```python
from build123d import *

# Parameters (mm, degrees)
F2_W           = 1
F2_H           = 12
F4_R           = 1.9571428571
F7_START       = 17.5
F7_DEPTH       = 42.5
F11_R          = 6
F12_DEPTH      = 25
F12_DEPTH_BACK = 25


with BuildPart() as f1:
    # F0 (on Front) → F1 (revolve)
    with BuildSketch(Plane.XZ):
        with BuildLine():
            Line((-199.1, 17.5), (-199.1, 0))
            Line((-199.1, 0), (75.9, 0))
            Line((75.9, 0), (75.9, 12.5))
            Line((75.9, 12.5), (70.9, 17.5))
            Line((70.9, 17.5), (26.1, 17.5))
            Line((26.1, 17.5), (26.1, 22.5))
            Line((26.1, 22.5), (22.4, 22.5))
            ThreePointArc((22.4, 22.5), (19.5715728753, 23.6715728753), (18.4, 26.5))
            Line((18.4, 26.5), (18.4, 30))
            Line((18.4, 30), (0, 30))
            Line((0, 30), (0, 22.5))
            Line((0, 22.5), (-69.7, 22.5))
            Line((-69.7, 22.5), (-69.7, 17.5))
            Line((-69.7, 17.5), (-199.1, 17.5))
        make_face()
    revolve(axis=Axis((-55.8219029194, 0, 0), (1, 0, 0)))

    # F2 (on Front) → F3 (revolve, cut)
    with BuildSketch(Plane.XZ):
        with Locations((-50.5, 27.5)):
            Rectangle(F2_W, F2_H)
    revolve(axis=Axis((-55.8219029194, 0, 0), (1, 0, 0)), mode=Mode.SUBTRACT)

    # F4 (on Front) → F5 (revolve, cut)
    with BuildSketch(Plane.XZ):
        with Locations((-86.2, 18.7571428571)):
            Circle(F4_R)
        with Locations((42.6, 18.7571428571)):
            Circle(F4_R)
        with BuildLine():
            Line((-3.4571428571, 32.4009352645), (-3.4571428571, 23.7571428571))
            ThreePointArc((-3.4571428571, 23.7571428571), (-2.1688399949, 21.9178328712), (0, 22.5))
            Line((0, 22.5), (0, 32.4009352645))
            Line((0, 32.4009352645), (-3.4571428571, 32.4009352645))
        make_face()
    revolve(axis=Axis((-55.8219029194, 0, 0), (1, 0, 0)), mode=Mode.SUBTRACT)

    # F6 (on Top) → F7 (cut)
    with BuildSketch(Plane.XY.offset(F7_START)):
        with BuildLine():
            Line((-9, 5), (-39, 5))
            ThreePointArc((-39, 5), (-44, 0), (-39, -5))
            Line((-39, -5), (-9, -5))
            ThreePointArc((-9, -5), (-4, 0), (-9, 5))
        make_face()
    extrude(amount=F7_DEPTH, mode=Mode.SUBTRACT)

    # F11 (on line) → F12 (cut, two sides)
    with BuildSketch(Plane(origin=(0, 0, 0), x_dir=(1, 0, 0), z_dir=(0, -0.8660254038, -0.5))) as f12_sk:
        with Locations((-149.1, 0)):
            Circle(F11_R)
    extrude(amount=-F12_DEPTH, mode=Mode.SUBTRACT)
    extrude(f12_sk.sketch, amount=F12_DEPTH_BACK, mode=Mode.SUBTRACT)


solid = f1.part
```
Input: part model. Units: mm. Frame: model coordinates. A direction names the side the tool comes from. Coordinates: 2 decimals unless noted, no trailing zeros. Write each loop counter-clockwise with the first axis right and the second up, starting at its lowest first coordinate (ties: lowest second). Pieces come first, ordered by that corner, then holes. Notation, with made-up numbers: (-14, 81.25) - (10, 81.25) arc R17 cw to (10, 111.25) - close; hole circle Ø2 at (36.25, 16.25). An arc over 180 degrees is marked (long way). Put each result on its own line as item: value. Start each with the question number.
1) Contact query for flat-ended pins moving along their axis: pin 1 (10 mm diameter, centred on x = -14.5, z = 4, fed in from +Y); pin 2 (5 mm diameter, centred on x = -10, y = -12.5, fed in from +Z); pin 3 (8 mm diameter, centred on x = 37, y = 22, fed in from +Z); pin 4 (6 mm diameter, centred on x = -168, z = -9, fed in from -Y). Output: stop coordinate, or through.
2) Reachability of faces 1 (the face through (-24, 5, 20)), 2 (the face through (26.1, 13, -12)), 3 (the face through (-50.493, -21.317, -2.799)), 4 (the face through (-144.18, -11.827, -12.898)), 5 (the face through (75.9, 0, 0)) from +Z, -Z, +X, -X, +Y, -Y: full face, straight path, thin tool, end or side. Return the list, or none.
3) Ray query, L1, parallel to X at y = 13, z = 3; L2, parallel to Z at x = -166, y = 0; L3, parallel to Z at x = -142.5, y = -12.5. Return the intervals inside material, ascending.
4) Cut plane A-A (x = -15). Return the cut outline in (y, z).
5) Mould query, pull axis X, two halves, no side actions, for faces 6 (the face through (-50, 2, -22)), 7 (the face through (33.495, 10.648, -13.887)), 8 (the face through (-24, -5, 20)), 9 (the face through (18.4, 27, 0)). Classes: pulls with the +X half, pulls with the -X half, needs draft (parallel to the pull), parting line crosses it, or undercut.
6) Cut plane B-B (x = -176.5). Return the cut outline in (y, z).
Resolved:
1. pin 1: stops at y = 22.5
1. pin 2: stops at z = 20.16
1. pin 3: passes through
1. pin 4: stops at y = -16.44
2. face 1: +Z
2. face 2: +X
2. face 3: none
2. face 4: -X
2. face 5: +Z, -Z, +X, +Y, -Y
3. L1: x = -199.1 to -153.66, -144.54 to 75.06
3. L2: z = -17.5 to 17.5
3. L3: z = -12.25 to 12.25
4. outline: (-5, 17.5) - (-5, 21.94) arc R22.5 ccw (long way) to (5, 21.94) - (5, 17.5) - close
5. face 6: undercut
5. face 7: needs draft
5. face 8: undercut
5. face 9: pulls with the +X half
6. outline: circle Ø35 at (0, 0)
